Build history of the part. All positions in model axes, mm. Face numbers are marked on the shaded views. A direction names the side the tool comes from. Give positions to 0.01 mm unless a question says otherwise; leave off trailing zeros. Order: outer loops, then holes, each group sorted by start corner. A loop starts at its lowest first (then second) coordinate and runs counter-clockwise, first axis right, second up. Notation, with made-up numbers: (70.5, 39.5) - (92.5, 39.5) arc R23 ccw to (92.5, 72.5) - close; hole circle Ø9 at (-4, 44.25). An arc over 180 degrees is marked (long way). Answer in a Markdown table with one row per item.
```python
from build123d import *

# Parameters (mm, degrees)
EXTRUDE_1_DEPTH     = 10
CUT_EXTRUDE_1_REACH = 13.95
SKETCH_2_R          = 2.58


with BuildPart() as part:
    # 草图1 → 凸台-拉伸1 (new body)
    with BuildSketch(Plane.XY):
        Polygon((-3, 0), (3, 0), (3, -1), (4.75, -1), (4.75, -3.251737131), (3, -4.5), (-3, -4.5), (-4.75, -3.251737131), (-4.75, -1), (-3, -1), align=None)
    extrude(amount=EXTRUDE_1_DEPTH)

    # 草图2 → 切除-拉伸1 (cut, up to next)
    with BuildSketch(Plane(origin=(0, 0, 0), x_dir=(1, 0, 0), z_dir=(0, 1, 0)), mode=Mode.PRIVATE) as cut_extrude_1_sk1:
        with Locations(Location((0, -5, 0), (0, 0, 270))):
            Circle(SKETCH_2_R)
    cut_extrude_1_tool1 = extrude(cut_extrude_1_sk1.sketch, amount=-CUT_EXTRUDE_1_REACH, mode=Mode.PRIVATE) & part.part
    add(cut_extrude_1_tool1.solids().sort_by_distance((0, 0, 5))[0], mode=Mode.SUBTRACT)


solid = part.part
```
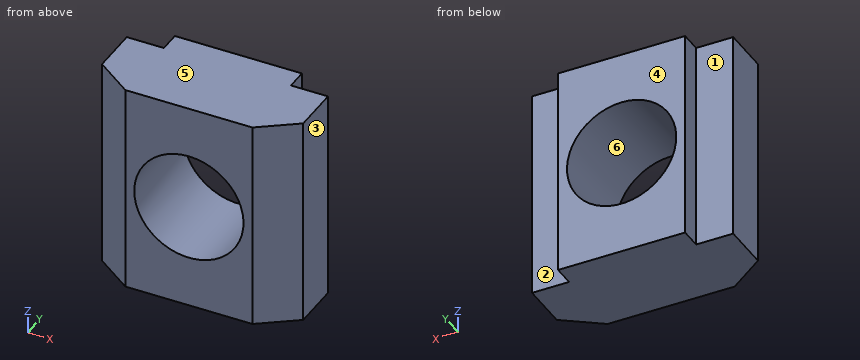
1. Drop flat-ended pins along their axis: P1, Ø4, axis at x = 0, z = 5, coming from the -Y side; P2, Ø0.9, axis at x = 4.5, z = 4, coming from the +Y side. Give the stop position or say it passes through.
Check result:
| item | result |
|---|---|
| P1 | passes through |
| P2 | stops at y = -1 |
2. Which spindle directions (+Z, -Z, +X, -X, +Y, -Y) get a long thin tool onto all of the face, cutting with end or side? Do the marked faces 1, 2 and 3. Say none if no direction does.
Check result:
| item | result |
|---|---|
| face 1 | +Z, -Z, -X, +Y |
| face 2 | +Z, -Z, +X, +Y |
| face 3 | +Z, -Z, +X, +Y, -Y |
3. Cut at D-D on x = 1. Write the cut outline in (y, z).
Check result:
| item | result |
|---|---|
| outline | (-4.5, 0) - (0, 0) - (0, 2.62) - (-4.5, 2.62) - close; (-4.5, 7.38) - (0, 7.38) - (0, 10) - (-4.5, 10) - close |
4. Cut at A-A on x = 0. Write the cut outline in (y, z), and give its area (3 significant figures).
Check result:
| item | result |
|---|---|
| outline | (-4.5, 0) - (0, 0) - (0, 2.42) - (-4.5, 2.42) - close; (-4.5, 7.58) - (0, 7.58) - (0, 10) - (-4.5, 10) - close |
| area | 21.8 mm² |
5. Two-plate mould, pull along Z, no slides. Class the marked faces 4, 5 and 6: +Z half, -Z half, draft (parallel to the pull), parting line (faces both ways), or undercut.
Check result:
| item | result |
|---|---|
| face 4 | draft |
| face 5 | +Z half |
| face 6 | undercut |
6. Cut at B-B on z = 5. Write the cut outline in (x, y), and give its area (3 significant figures).
Check result:
| item | result |
|---|---|
| outline | (-4.75, -3.25) - (-3, -4.5) - (-2.58, -4.5) - (-2.58, 0) - (-3, 0) - (-3, -1) - (-4.75, -1) - close; (2.58, -4.5) - (3, -4.5) - (4.75, -3.25) - (4.75, -1) - (3, -1) - (3, 0) - (2.58, 0) - close |
| area | 13.8 mm² |
7. Probe line 1 (X direction, y = -1.5, z = 5); line 2 (X direction, y = -3.1, z = 7); line 3 (Z direction, x = 2.25, y = -1.1). List the from-to ranges inside material, lowest first.
Check result:
| item | result |
|---|---|
| line 1 | x = -4.75 to -2.58, 2.58 to 4.75 |
| line 2 | x = -4.75 to -1.63, 1.63 to 4.75 |
| line 3 | z = 0 to 3.74, 6.26 to 10 |
8. Cut at C-C on y = -0.7. Write the cut outline in (x, z).
Check result:
| item | result |
|---|---|
| outline | (-3, 0) - (3, 0) - (3, 10) - (-3, 10) - close; hole circle Ø5.16 at (0, 5) |
